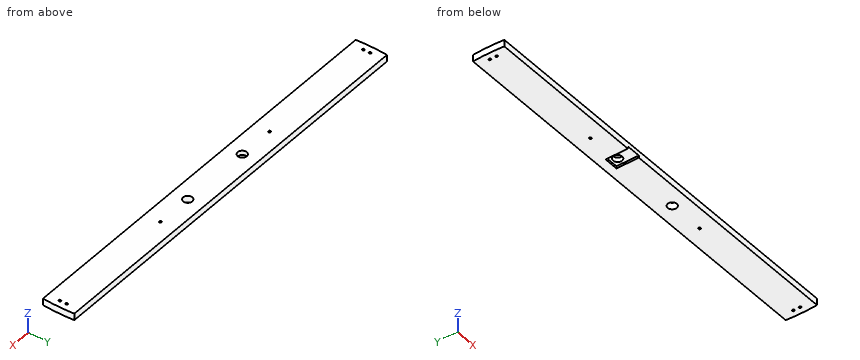
from build123d import *

# Parameters (mm, degrees)
SKETCH1_R           = 12.7
SKETCH1_R_2         = 3.175
BOSS_EXTRUDE2_DEPTH = 19.05
SKETCH2_W           = 40.64
SKETCH2_H           = 127
CUT_EXTRUDE1_DEPTH  = 6.35


with BuildPart() as part:
    # Sketch1 → Boss-Extrude2 (new body)
    with BuildSketch(Plane.XY):
        with BuildLine():
            Line((582.506512839, 44.45), (-582.506512839, 44.45))
            ThreePointArc((-582.506512839, 44.45), (-584.2, 0), (-582.506512839, -44.45))
            Line((-582.506512839, -44.45), (582.506512839, -44.45))
            ThreePointArc((582.506512839, -44.45), (584.2, 0), (582.506512839, 44.45))
        make_face()
        with Locations(Location((101.6, 0, 0), (0, 0, 180))):
            Circle(SKETCH1_R, mode=Mode.SUBTRACT)
        with Locations(Location((-565.069727445, 9.525, 0), (0, 0, 180))):
            Circle(SKETCH1_R_2, mode=Mode.SUBTRACT)
        with Locations(Location((-565.069727445, -9.525, 0), (0, 0, 180))):
            Circle(SKETCH1_R_2, mode=Mode.SUBTRACT)
        with Locations(Location((565.069727445, -9.525, 0), (0, 0, 180))):
            Circle(SKETCH1_R_2, mode=Mode.SUBTRACT)
        with Locations(Location((565.069727445, 9.525, 0), (0, 0, 180))):
            Circle(SKETCH1_R_2, mode=Mode.SUBTRACT)
        with Locations(Location((-101.6, 0, 0), (0, 0, 180))):
            Circle(SKETCH1_R, mode=Mode.SUBTRACT)
        with Locations(Location((-203.2, 0, 0), (0, 0, 180))):
            Circle(SKETCH1_R_2, mode=Mode.SUBTRACT)
        with Locations(Location((203.2, 0, 0), (0, 0, 180))):
            Circle(SKETCH1_R_2, mode=Mode.SUBTRACT)
    extrude(amount=BOSS_EXTRUDE2_DEPTH)

    # Sketch2 → Cut-Extrude1 (cut)
    with BuildSketch(Plane.XY):
        with Locations((-101.6, -44.45)):
            Rectangle(SKETCH2_W, SKETCH2_H)
    extrude(amount=CUT_EXTRUDE1_DEPTH, mode=Mode.SUBTRACT)


solid = part.part
Here's how the part is built. I have some questions about the finished solid (model axes, mm). Coordinates: 2 decimals unless noted, no trailing zeros. Loops run counter-clockwise (first coordinate to the right, second up) from the corner with the lowest first, then second, coordinate; pieces in that order, holes last.
1. For P1, Ø10, axis at x = 565.07, y = -9.52, coming from the +Z side; P2, Ø10, axis at y = -19, z = 10, coming from the +X side; P3, Ø5, axis at x = 203.2, y = 0, coming from the +Z side, each with a flat end and sliding along its axis, tell me the tip position at first contact or that it passes through.
2. Imagine slicing it at B-B, the plane z = 3. Please give me the cut outline in (x, y) (3 decimals), and give its area (3 significant figures).
3. Imagine slicing it at A-A, the plane x = 101.6. Please give me the cut outline in (y, z), and give its area (3 significant figures).
4. I need wall thicknesses on L1, parallel to X at y = 14, z = 10.5; L2, parallel to Y at x = 203.2, z = 6.75 (3 decimals); L3, parallel to X at y = -38.5, z = 1. Which ranges of each line are inside material? Lowest first, please.
Taken from the geometry:
1. P1: stops at z = 19.05
1. P2: stops at x = 584.03
1. P3: passes through
2. outline: (-582.507, -44.45) - (-121.92, -44.45) - (-121.92, 19.05) - (-81.28, 19.05) - (-81.28, -44.45) - (582.507, -44.45) arc R584.2 ccw to (582.507, 44.45) - (-582.507, 44.45) arc R584.2 ccw to start; hole circle Ø6.35 at (-565.07, -9.525); hole circle Ø6.35 at (-565.07, 9.525); hole circle Ø6.35 at (-203.2, 0); hole circle Ø25.4 at (101.6, 0); hole circle Ø6.35 at (203.2, 0); hole circle Ø6.35 at (565.07, -9.525); hole circle Ø6.35 at (565.07, 9.525)
2. area: 100,000 mm2
3. outline: (-44.45, 0) - (-12.7, 0) - (-12.7, 19.05) - (-44.45, 19.05) - close; (12.7, 0) - (44.45, 0) - (44.45, 19.05) - (12.7, 19.05) - close
3. area: 1,210 mm2
4. L1: x = -584.03 to 584.03
4. L2: y = -44.45 to -3.175, 3.175 to 44.45
4. L3: x = -582.93 to -121.92, -81.28 to 582.93
